```python
from build123d import *

# Parameters (mm, degrees)
F0_R     = 4
F1_DEPTH = 2.5
F2_R     = 20


with BuildPart() as f1:
    # F0 (on Top) → F1 (new body, symmetric)
    with BuildSketch(Plane.XY):
        with BuildLine():
            Line((38.5, -75), (75, -75))
            Line((75, -75), (75, 75))
            Line((75, 75), (38.5, 75))
            ThreePointArc((38.5, 75), (0, 36.5), (-38.5, 75))
            Line((-38.5, 75), (-75, 75))
            Line((-75, 75), (-75, -75))
            Line((-75, -75), (-38.5, -75))
            ThreePointArc((-38.5, -75), (0, -36.5), (38.5, -75))
        make_face()
        with Locations((-55, -55)):
            Circle(F0_R, mode=Mode.SUBTRACT)
        with Locations((55, -55)):
            Circle(F0_R, mode=Mode.SUBTRACT)
        with Locations((-55, 55)):
            Circle(F0_R, mode=Mode.SUBTRACT)
        with Locations((55, 55)):
            Circle(F0_R, mode=Mode.SUBTRACT)
    extrude(amount=F1_DEPTH, both=True)

    # F2
    f2_edges = [f1.edges().sort_by_distance(p)[0] for p in [
        (75, -75, 0),
        (75, 75, 0),
        (-75, 75, 0),
        (-38.5, 75, 0),
        (38.5, 75, 0),
        (-38.5, -75, 0),
        (38.5, -75, 0),
        (-75, -75, 0),
    ]]
    fillet(f2_edges, radius=F2_R)


solid = f1.part
```
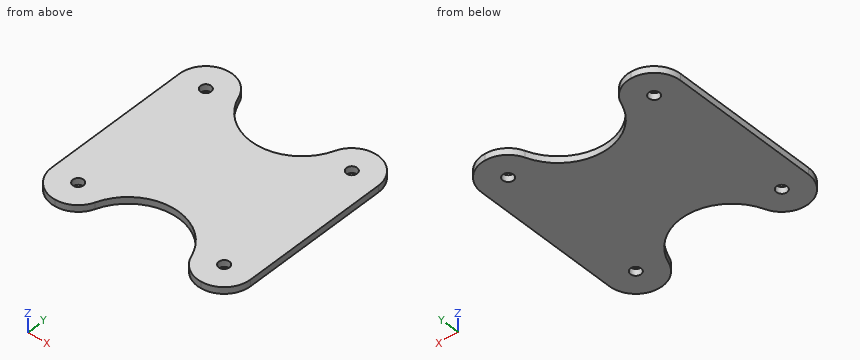
The model under review builds one solid part; all positions refer to its coordinate system, in mm. Round coordinates to 2 decimals unless told otherwise and drop trailing zeros. Loops run counter-clockwise (first coordinate to the right, second up) from the corner with the lowest first, then second, coordinate; pieces in that order, holes last.
1) Consider section B-B on y = -43. State the section outline as (x, z) points.
Values follow:
outline: (-75, -2.5) - (-21.41, -2.5) - (-21.41, 2.5) - (-75, 2.5) - close; (21.41, -2.5) - (75, -2.5) - (75, 2.5) - (21.41, 2.5) - close
2) Clearance check with a flat-ended pin moving along its axis: P1, Ø3, axis at x = 57, z = -2, coming from the -Y side. State where the tip first meets the part, or that it passes through.
Values follow:
P1: stops at y = -74.99
3) Consider section D-D on x = -9. State the section outline as (y, z) points.
Values follow:
outline: (-37.57, -2.5) - (37.57, -2.5) - (37.57, 2.5) - (-37.57, 2.5) - close
4) Wall thickness on line 1 along Y through (x, z) = (55, -1.15); line 2 along X through (y, z) = (-54.5, 0.7); line 3 along X through (y, z) = (-44.5, 1.95): over which ranges is each line inside the solid? List them lowest first.
Values follow:
line 1: y = -75 to -59, -51 to 51, 59 to 75
line 2: x = -75 to -58.97, -51.03 to -32.59, 32.59 to 51.03, 58.97 to 75
line 3: x = -75 to -23.49, 23.49 to 75
5) Consider section A-A on z = 0.45. State the section outline as (x, y) points (3 decimals).
Values follow:
outline: (-75, -55) arc R20 ccw to (-55, -75) - (-54.975, -75) arc R20 ccw to (-36.18, -61.838) arc R38.5 cw to (36.18, -61.838) arc R20 ccw to (54.975, -75) - (55, -75) arc R20 ccw to (75, -55) - (75, 55) arc R20 ccw to (55, 75) - (54.975, 75) arc R20 ccw to (36.18, 61.838) arc R38.5 cw to (-36.18, 61.838) arc R20 ccw to (-54.975, 75) - (-55, 75) arc R20 ccw to (-75, 55) - close; hole circle Ø8 at (-55, -55); hole circle Ø8 at (-55, 55); hole circle Ø8 at (55, -55); hole circle Ø8 at (55, 55)
6) Consider section C-C on y = 64.5. State the section outline as (x, z) points, then the cut area to 3 significant figures.
Values follow:
outline: (-72.6, -2.5) - (-37.38, -2.5) - (-37.38, 2.5) - (-72.6, 2.5) - close; (37.38, -2.5) - (72.6, -2.5) - (72.6, 2.5) - (37.38, 2.5) - close
area: 352 mm2
